Design review of the part built by this model. Coordinates are the model's own, in mm. A direction names the side the tool comes from. Coordinates: 2 decimals unless noted, no trailing zeros. Write each loop counter-clockwise with the first axis right and the second up, starting at its lowest first coordinate (ties: lowest second). Pieces come first, ordered by that corner, then holes. Notation, with made-up numbers: (13.5, -4) - (29.5, -4) arc R22 ccw to (29.5, 2) - close; hole circle Ø5 at (89, 37.5). An arc over 180 degrees is marked (long way). Use a Markdown table: item, result.
from build123d import *

# Parameters (mm, degrees)
SKETCH2_R                    = 22.5
SKETCH2_R_2                  = 12.3
SKETCH2_R_3                  = 1.25
SKETCH2_R_4                  = 1.5
BOSS_EXTRUDE1_DEPTH          = 5
CUT_EXTRUDE1_DEPTH           = 2.5
CIRPATTERN1_COUNT            = 3
SKETCH4_R                    = 3.3
SKETCH4_R_2                  = 2.5
BOSS_EXTRUDE2_DEPTH          = 1.5
FILLET1_R                    = 1.5
CHAMFER1_SIZE                = 0.25
CIRPATTERN2_COUNT            = 3
FILLET1_OF_CIRPATTERN2_R     = 1.5
CHAMFER1_OF_CIRPATTERN2_SIZE = 0.25


with BuildPart() as part:
    # Sketch2 → Boss-Extrude1 (new body)
    with BuildSketch(Plane.XY):
        Circle(SKETCH2_R)
        Circle(SKETCH2_R_2, mode=Mode.SUBTRACT)
        with Locations((0, 17.1)):
            Circle(SKETCH2_R_3, mode=Mode.SUBTRACT)
        with Locations((14.809034405, -8.55)):
            Circle(SKETCH2_R_3, mode=Mode.SUBTRACT)
        with Locations((16.02146997, 9.25)):
            Circle(SKETCH2_R_4, mode=Mode.SUBTRACT)
        with Locations((0, -18.5)):
            Circle(SKETCH2_R_4, mode=Mode.SUBTRACT)
        with Locations((-14.809034405, -8.55)):
            Circle(SKETCH2_R_3, mode=Mode.SUBTRACT)
        with Locations((-16.02146997, 9.25)):
            Circle(SKETCH2_R_4, mode=Mode.SUBTRACT)
    extrude(amount=BOSS_EXTRUDE1_DEPTH)

    # Sketch3 → Cut-Extrude1 (cut)
    with BuildSketch(Plane.XY.offset(5)):
        Polygon((-2.886751346, 17.1), (-1.443375673, 14.6), (1.443375673, 14.6), (2.886751346, 17.1), (1.443375673, 19.6), (-1.443375673, 19.6), align=None)
        Polygon((16.02146997, 6.074573519), (18.77146997, 7.66228676), (18.77146997, 10.83771324), (16.02146997, 12.425426481), (13.27146997, 10.83771324), (13.27146997, 7.66228676), align=None)
    cut_extrude1 = extrude(amount=-CUT_EXTRUDE1_DEPTH, mode=Mode.SUBTRACT)

    # CirPattern1: Cut-Extrude1 ×3 about axis
    cirpattern1_axis = Axis((0, 0, 0), (0, 0, 1))
    for i in range(1, CIRPATTERN1_COUNT):
        add(cut_extrude1.rotate(cirpattern1_axis, i * 360 / CIRPATTERN1_COUNT), mode=Mode.SUBTRACT)

    # Sketch4 → Boss-Extrude2 (add)
    with BuildSketch(Plane(origin=(0, 0, 0), x_dir=(-1, 0, 0), z_dir=(0, 0, -1))):
        with Locations(Location((0, 17.1, 0), (0, 0, 180))):
            Circle(SKETCH4_R)
        with Locations((0, 17.1)):
            Circle(SKETCH4_R_2, mode=Mode.SUBTRACT)
    boss_extrude2 = extrude(amount=BOSS_EXTRUDE2_DEPTH)

    # Fillet1
    fillet1_edges = [part.edges().sort_by_distance(p)[0] for p in [
        (-3.3, 17.1, 0),
    ]]
    fillet(fillet1_edges, radius=FILLET1_R - 0.0001)  # a hair under: the kernel refuses the full size

    # Chamfer1
    chamfer1_edges = [part.edges().sort_by_distance(p)[0] for p in [
        (2.5, 17.1, -1.5),
    ]]
    chamfer(chamfer1_edges, length=CHAMFER1_SIZE)

    # CirPattern2: Boss-Extrude2 ×3 about axis
    cirpattern2_axis = Axis((0, 0, 0), (0, 0, 1))
    for i in range(1, CIRPATTERN2_COUNT):
        add(boss_extrude2.rotate(cirpattern2_axis, i * 360 / CIRPATTERN2_COUNT))

    # Fillet1 of CirPattern2
    fillet1_of_cirpattern2_edges = [part.edges().sort_by_distance(p)[0] for p in [
        (-13.159034405, -11.407883832, 0),
        (16.459034405, -5.692116168, 0),
    ]]
    fillet(fillet1_of_cirpattern2_edges, radius=FILLET1_OF_CIRPATTERN2_R - 0.0001)  # a hair under: the kernel refuses the full size

    # Chamfer1 of CirPattern2
    chamfer1_of_cirpattern2_edges = [part.edges().sort_by_distance(p)[0] for p in [
        (-16.059034405, -6.384936491, -1.5),
        (13.559034405, -10.715063509, -1.5),
    ]]
    chamfer(chamfer1_of_cirpattern2_edges, length=CHAMFER1_OF_CIRPATTERN2_SIZE)


solid = part.part
(1) Take a section at C-C on y = 9.25. Write out the cut boundary in (x, z).
Determined:
| item | result |
|---|---|
| outline | (-20.51, 0) - (-17.52, 0) - (-17.52, 2.5) - (-18.77, 2.5) - (-18.77, 5) - (-20.51, 5) - close; (-14.52, 0) - (-8.11, 0) - (-8.11, 5) - (-13.27, 5) - (-13.27, 2.5) - (-14.52, 2.5) - close; (8.11, 0) - (14.52, 0) - (14.52, 2.5) - (13.27, 2.5) - (13.27, 5) - (8.11, 5) - close; (17.52, 0) - (20.51, 0) - (20.51, 5) - (18.77, 5) - (18.77, 2.5) - (17.52, 2.5) - close |
(2) Draft analysis for pull direction Y (two halves, no side actions). For faces 4 (the flat face through (-15, -7, 2.5)), 5 (the flat face through (-2, 15, -1.5)), state which applies: +Y half, -Y half, draft (parallel to the pull), parting line (faces both ways), or undercut.
Determined:
| item | result |
|---|---|
| face 4 | undercut |
| face 5 | draft |
(3) For pin 1 (1.2 mm diameter, centred on y = 9, z = 3.5, fed in from -X); pin 2 (4 mm diameter, centred on x = -14.81, y = -8.55, fed in from +Z); pin 3 (1.2 mm diameter, centred on y = -18.5, z = 4, fed in from -X), all flat-tipped, find the tip position at first contact; note any pin that passes through.
Determined:
| item | result |
|---|---|
| pin 1 | x = -20.87 |
| pin 2 | z = 2.5 |
| pin 3 | x = -13.63 |
(4) For L1, parallel to Y at x = 0, z = 1.75; L2, parallel to Y at x = 1.5, z = 4.5; L3, parallel to X at y = -8.55, z = 0.5, list the stretches that pass through material, from the lowest coordinate up. Write a range as from..to.
Determined:
| item | result |
|---|---|
| L1 | -22.5..-20, -17..-12.3, 12.3..15.85, 18.35..22.5 |
| L2 | -22.45..-20.81, -16.19..-12.21, 12.21..14.7, 19.5..22.45 |
| L3 | -20.81..-16.06, -13.56..-8.84, 8.84..13.56, 16.06..20.81 |
(5) Take a section at A-A on y = 0. Write out the cut boundary in (x, z).
Determined:
| item | result |
|---|---|
| outline | (-22.5, 0) - (-12.3, 0) - (-12.3, 5) - (-22.5, 5) - close; (12.3, 0) - (22.5, 0) - (22.5, 5) - (12.3, 5) - close |
(6) Take a section at D-D on y = -18.5. Write out the cut boundary in (x, z), and give its area (3 significant figures).
Determined:
| item | result |
|---|---|
| outline | (-12.81, 0) - (-1.5, 0) - (-1.5, 2.5) - (-2.75, 2.5) - (-2.75, 5) - (-12.81, 5) - close; (1.5, 0) - (12.81, 0) - (12.81, 5) - (2.75, 5) - (2.75, 2.5) - (1.5, 2.5) - close |
| area | 107 mm2 |
(7) Take a section at B-B on x = -9. Write out the cut boundary in (y, z), and give its area (3 significant figures).
Determined:
| item | result |
|---|---|
| outline | (-20.62, 0) - (-8.38, 0) - (-8.38, 5) - (-20.62, 5) - close; (8.38, 0) - (20.62, 0) - (20.62, 5) - (8.38, 5) - close |
| area | 122 mm2 |
(8) Machinability: for faces 1 (the cylindrical face through (14.523, 9.316, 1.232)), 2 (the cylindrical face through (-1.34, 19.21, -0.62)), 3 (the flat face through (-14.63, 11.62, 3.77)), which of the approach directions +Z, -Z, +X, -X, +Y, -Y give a long, thin tool a straight path to every point of the face, cutting with its end or side? Answer none if there is none.
Determined:
| item | result |
|---|---|
| face 1 | +Z, -Z |
| face 2 | -Z |
| face 3 | +Z |
